from build123d import *

# Parameters (mm, degrees)
F0_R       = 6.35
F0_R_2     = 2.159
F1_DEPTH   = 1.27
F2_R       = 6.35
F2_R_2     = 4.445
F3_DEPTH   = 15.875
F5_R       = 1.9939
F6_DEPTH   = 6.35
F7_COUNT   = 3
F8_R       = 1.9939
F6_FACE_R  = 1.9939
F9_DEPTH   = 6.35
F7_FACE_R  = 1.9939
F10_R      = 1.9939
F11_DEPTH  = 6.35
F7_FACE1_R = 1.9939
F12_R      = 1.9939
F13_DEPTH  = 6.35


with BuildPart() as f1:
    # F0 (on Top) → F1 (new body)
    with BuildSketch(Plane.XY):
        Circle(F0_R)
        Circle(F0_R_2, mode=Mode.SUBTRACT)
    extrude(amount=F1_DEPTH)

    # F2 (on face) → F3 (join)
    with BuildSketch(Plane.XY.offset(1.27)):
        Circle(F2_R)
        Circle(F2_R_2, mode=Mode.SUBTRACT)
    extrude(amount=F3_DEPTH)


with BuildPart() as f6:
    # F5 (on offset) → F6 (new body)
    with BuildSketch(Plane.YZ.offset(6.35)):
        with Locations((0, 6.35)):
            Circle(F5_R)
    extrude(amount=-F6_DEPTH)


with BuildPart() as f6b:
    # F5 (on offset) → F6, piece 2 (new body)
    with BuildSketch(Plane.YZ.offset(6.35)):
        with Locations((0, 12.7)):
            Circle(F5_R)
    extrude(amount=-F6_DEPTH)


with BuildPart() as f7_1:
    # F7: instance of F6
    add(f6.part.rotate(Axis((0, 0, 17.145), (0, 0, 1)), 1 * 360 / F7_COUNT))


with BuildPart() as f7_2:
    # F7: instance of F6
    add(f6.part.rotate(Axis((0, 0, 17.145), (0, 0, 1)), 2 * 360 / F7_COUNT))


with BuildPart() as f7_3:
    # F7: instance of F6b
    add(f6b.part.rotate(Axis((0, 0, 17.145), (0, 0, 1)), 1 * 360 / F7_COUNT))


with BuildPart() as f7_4:
    # F7: instance of F6b
    add(f6b.part.rotate(Axis((0, 0, 17.145), (0, 0, 1)), 2 * 360 / F7_COUNT))


with BuildPart() as f9_tool:
    # F8 (on face) + F6_face (on face) → F9 (new body)
    with BuildSketch(Plane.YZ.offset(6.35)):
        with Locations((0, 6.35)):
            Circle(F8_R)
    with BuildSketch(Plane(origin=(6.35, 0, 6.35), x_dir=(0, 1, 0), z_dir=(1, 0, 0))):
        with Locations((0, 6.35)):
            Circle(F6_FACE_R)
    extrude(amount=-F9_DEPTH)


with BuildPart() as f1_1:
    add(f1.part)

    # F9: cut by f9_tool
    add(f9_tool.part, mode=Mode.SUBTRACT)


with BuildPart() as f6_1:
    add(f6.part)

    # F9: cut by f9_tool
    add(f9_tool.part, mode=Mode.SUBTRACT)


with BuildPart() as f6b_1:
    add(f6b.part)

    # F9: cut by f9_tool
    add(f9_tool.part, mode=Mode.SUBTRACT)


with BuildPart() as f7_1_1:
    add(f7_1.part)

    # F9: cut by f9_tool
    add(f9_tool.part, mode=Mode.SUBTRACT)


with BuildPart() as f7_2_1:
    add(f7_2.part)

    # F9: cut by f9_tool
    add(f9_tool.part, mode=Mode.SUBTRACT)


with BuildPart() as f7_3_1:
    add(f7_3.part)

    # F9: cut by f9_tool
    add(f9_tool.part, mode=Mode.SUBTRACT)


with BuildPart() as f7_4_1:
    add(f7_4.part)

    # F9: cut by f9_tool
    add(f9_tool.part, mode=Mode.SUBTRACT)


with BuildPart() as f11_tool:
    # F7_face (on face) + F10 (on face) → F11 (new body)
    with BuildSketch(Plane(origin=(-3.175, 5.499261314, 6.35), x_dir=(-0.8660254038, -0.5, 0), z_dir=(-0.5, 0.8660254038, 0))):
        with Locations((0, 6.35)):
            Circle(F7_FACE_R)
    with BuildSketch(Plane(origin=(-3.175, 5.499261314, 0), x_dir=(-0.8660254038, -0.5, 0), z_dir=(-0.5, 0.8660254038, 0))):
        with Locations((0, 6.35)):
            Circle(F10_R)
    extrude(amount=-F11_DEPTH)


with BuildPart() as f1_2:
    add(f1_1.part)

    # F11: cut by f11_tool
    add(f11_tool.part, mode=Mode.SUBTRACT)


with BuildPart() as f7_1_2:
    add(f7_1_1.part)

    # F11: cut by f11_tool
    add(f11_tool.part, mode=Mode.SUBTRACT)


with BuildPart() as f7_2_2:
    add(f7_2_1.part)

    # F11: cut by f11_tool
    add(f11_tool.part, mode=Mode.SUBTRACT)


with BuildPart() as f7_3_2:
    add(f7_3_1.part)

    # F11: cut by f11_tool
    add(f11_tool.part, mode=Mode.SUBTRACT)


with BuildPart() as f7_4_2:
    add(f7_4_1.part)

    # F11: cut by f11_tool
    add(f11_tool.part, mode=Mode.SUBTRACT)


with BuildPart() as f13_tool:
    # F7_face1 (on face) + F12 (on face) → F13 (new body)
    with BuildSketch(Plane(origin=(-3.175, -5.499261314, 6.35), x_dir=(0.8660254038, -0.5, 0), z_dir=(-0.5, -0.8660254038, 0))):
        with Locations((0, 6.35)):
            Circle(F7_FACE1_R)
    with BuildSketch(Plane(origin=(-3.175, -5.499261314, 0), x_dir=(0.8660254038, -0.5, 0), z_dir=(-0.5, -0.8660254038, 0))):
        with Locations((0, 6.35)):
            Circle(F12_R)
    extrude(amount=-F13_DEPTH)


with BuildPart() as f1_3:
    add(f1_2.part)

    # F13: cut by f13_tool
    add(f13_tool.part, mode=Mode.SUBTRACT)


with BuildPart() as f7_2_3:
    add(f7_2_2.part)

    # F13: cut by f13_tool
    add(f13_tool.part, mode=Mode.SUBTRACT)


with BuildPart() as f7_4_3:
    add(f7_4_2.part)

    # F13: cut by f13_tool
    add(f13_tool.part, mode=Mode.SUBTRACT)


solid = f1_3.part
Check sheet for the modelled part. Datum: model origin and axes. Units: mm. A direction names the side the tool comes from. Coordinates: 2 decimals unless noted, no trailing zeros. Write each loop counter-clockwise with the first axis right and the second up, starting at its lowest first coordinate (ties: lowest second). Pieces come first, ordered by that corner, then holes. Notation, with made-up numbers: M 64,-33.75 L 81,-33.75 A26 cw 81,3.25 Z; hole C -34.5,-16.75 d6. An arc over 180 degrees is marked long. Answer as CSV lines item,"result".
Q1. Cross-section at A-A (y = 0). Record the boundary of the cut face in (x, z) (3 decimals).
Check result:
outline,"M -6.35,0 L -2.159,0 L -2.159,1.27 L -4.445,1.27 L -4.445,17.145 L -6.35,17.145 Z; M 2.159,0 L 6.35,0 L 6.35,4.356 L 4.445,4.356 L 4.445,1.27 L 2.159,1.27 Z; M 4.445,8.344 L 6.35,8.344 L 6.35,10.706 L 4.445,10.706 Z; M 4.445,14.694 L 6.35,14.694 L 6.35,17.145 L 4.445,17.145 Z"
Q2. Set-up check for faces 1 (the face through (5.18, 1.9, 6.95)), 2 (the face through (2.051, -3.943, 9.096)), 3 (the face through (-4.236, 3.534, 6.949)): record each of +Z, -Z, +X, -X, +Y, -Y from which the full face is reachable in a straight line by a thin tool's end or side.
Check result:
face 1,"+X"
face 2,"+Z"
face 3,"none"
Q3. Go/stop test with flat-tipped pins: pin 1 (1 mm diameter, centred on y = -1.5, z = 3, fed in from +X); pin 2 (3.5 mm diameter, centred on y = 0, z = 12.7, fed in from +X); pin 3 (6 mm diameter, centred on x = -1.5, y = 1.5, fed in from -Z); pin 4 (6 mm diameter, centred on x = 3.5, z = 2.5, fed in from -Y). Record where each tip stops, or that it passes through.
Check result:
pin 1,"x = 6.27"
pin 2,"x = -4.09"
pin 3,"z = 0"
pin 4,"y = -6.33"
Q4. Cross-section at D-D (x = 2.75). Record the boundary of the cut face in (y, z) (3 decimals), then the cut area to 3 significant figures.
Check result:
outline,"M -5.724,0 L 5.724,0 L 5.724,17.145 L 3.492,17.145 L 3.492,1.27 L -3.492,1.27 L -3.492,17.145 L -5.724,17.145 Z"
area,"85.4 mm^2"
Q5. Cross-section at C-C (z = 8). Record the boundary of the cut face in (x, y) (3 decimals).
Check result:
outline,"M -4.095,-4.853 L -3.12,-3.166 A4.445 cw -3.12,3.166 L -4.095,4.853 A6.35 ccw Z; M -2.156,-5.973 A6.35 ccw 6.251,-1.119 L 4.302,-1.119 A4.445 cw -1.181,-4.285 Z; M -2.156,5.973 L -1.181,4.285 A4.445 cw 4.302,1.119 L 6.251,1.119 A6.35 ccw Z"
Q6. Cross-section at B-B (x = 0). Record the boundary of the cut face in (y, z) (3 decimals), then the cut area to 3 significant figures.
Check result:
outline,"M -6.35,0 L -2.159,0 L -2.159,1.27 L -4.445,1.27 L -4.445,17.145 L -6.35,17.145 Z; M 2.159,0 L 6.35,0 L 6.35,17.145 L 4.445,17.145 L 4.445,1.27 L 2.159,1.27 Z"
area,"71.1 mm^2"
Q7. Material ranges on probe 1 along Z at (x, y) = (5, 0) (3 decimals); probe 2 along Y at (x, z) = (0, 0.5); probe 3 along Z at (x, y) = (-2.25, 4.75) (3 decimals), recorded low to high. Write a range as from..to.
Check result:
probe 1,"0..4.356, 8.344..10.706, 14.694..17.145"
probe 2,"-6.35..-2.16, 2.16..6.35"
probe 3,"0..4.402, 8.298..10.752, 14.648..17.145"
Q8. Mould release check, pull along Z, two halves, no side actions. Record for faces 4 (the face through (5.178, 1.842, 11.936)), 5 (the face through (-0.28, 2.14, 0.63)), 6 (the face through (3, -4, 17.145)): released by +Z, released by -Z, zero draft, split by the parting line, or undercut.
Check result:
face 4,"undercut"
face 5,"zero draft"
face 6,"released by +Z"
